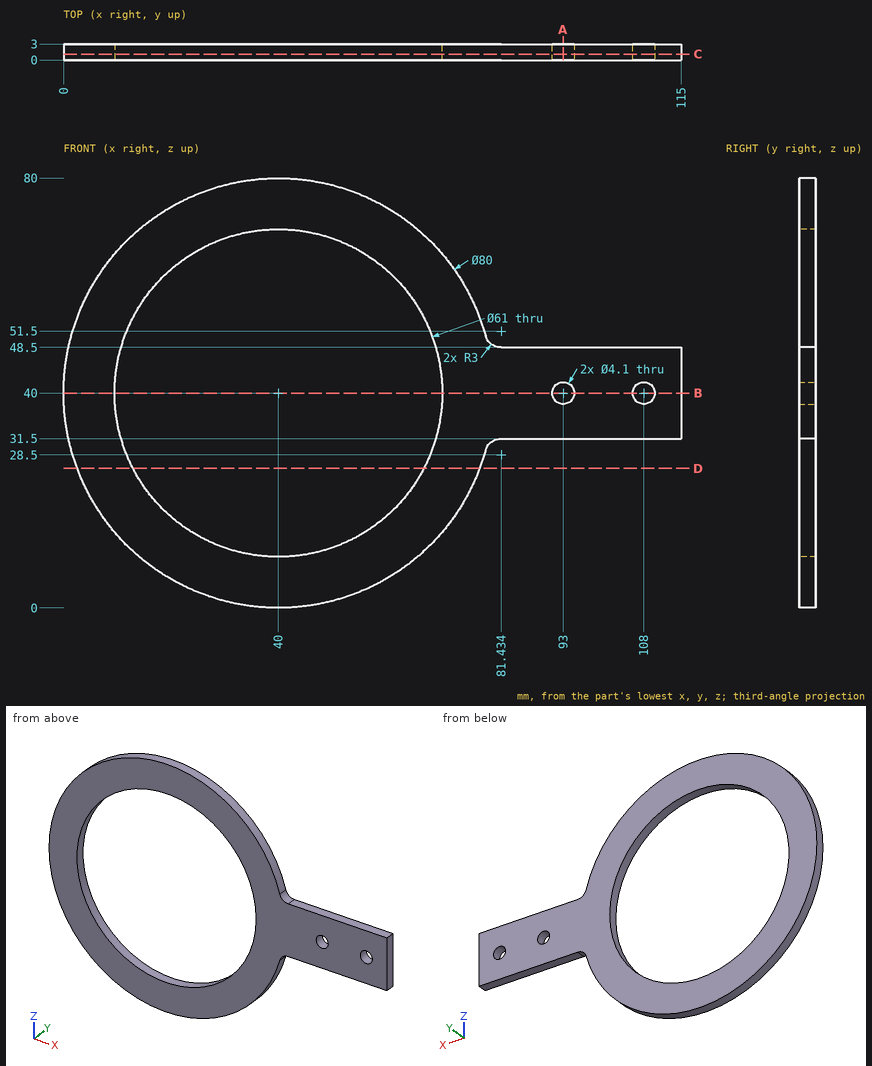
Input: dimensioned drawing with shaded views. Units: mm. Origin: part minimum x, y, z. Coordinates: 2 decimals unless noted, no trailing zeros. Loops run counter-clockwise (first coordinate to the right, second up) from the corner with the lowest first, then second, coordinate; pieces in that order, holes last. Notation, with made-up numbers: (-15, 78) -> (5, 78) arc R23 ccw to (5, 106) -> close; hole circle Ø8 at (-25, 13.5). An arc over 180 degrees is marked (long way). Use a Markdown table: item, result. Add a question column.
(1) Line query: line 1 along Z through (x, y) = (93, 1.75); line 2 along Z through (x, y) = (40, 2.3); line 3 along X through (y, z) = (0.55, 49.5) (1 decimal). Output: solid intervals per line, ascending.
(2) Section query A-A, the plane x = 93. Return loops of the section in (y, z), plus the area to 3 significant figures.
(3) Section query C-C, the plane y = 1.1. Return loops of the section in (x, z).
(4) Pin query (flat end, axial travel): pin 1 Ø1.5 at (x, y) = (23, 2) entering from -Z; pin 2 Ø0.9 at (x, y) = (101.5, 2) entering from -Z; pin 3 Ø4.5 at (x, z) = (93, 40) entering from -Y; pin 4 Ø2.5 at (x, z) = (108, 40) entering from -Y. Return the tip coordinate at first contact, or that it passes through.
(5) Section query B-B, the plane z = 40. Return loops of the section in (x, y), plus the area to 3 significant figures.
(6) Section query D-D, the plane z = 26. Return loops of the section in (x, y).
Answer:
| question | item | result |
|---|---|---|
| 1 | line 1 | z = 31.5 to 37.95, 42.05 to 48.5 |
| 1 | line 2 | z = 0 to 9.5, 70.5 to 80 |
| 1 | line 3 | x = 1.1 to 11, 69 to 79.2 |
| 2 | outline | (0, 31.5) -> (3, 31.5) -> (3, 37.95) -> (0, 37.95) -> close; (0, 42.05) -> (3, 42.05) -> (3, 48.5) -> (0, 48.5) -> close |
| 2 | area | 38.7 mm^2 |
| 3 | outline | (78.54, 29.3) arc R3 cw to (81.43, 31.5) -> (115, 31.5) -> (115, 48.5) -> (81.43, 48.5) arc R3 cw to (78.54, 50.7) arc R40 ccw (long way) to start; hole circle Ø61 at (40, 40); hole circle Ø4.1 at (93, 40); hole circle Ø4.1 at (108, 40) |
| 4 | pin 1 | stops at z = 3.45 |
| 4 | pin 2 | stops at z = 31.5 |
| 4 | pin 3 | stops at y = 0 |
| 4 | pin 4 | passes through |
| 5 | outline | (0, 0) -> (9.5, 0) -> (9.5, 3) -> (0, 3) -> close; (70.5, 0) -> (90.95, 0) -> (90.95, 3) -> (70.5, 3) -> close; (95.05, 0) -> (105.95, 0) -> (105.95, 3) -> (95.05, 3) -> close; (110.05, 0) -> (115, 0) -> (115, 3) -> (110.05, 3) -> close |
| 5 | area | 137 mm^2 |
| 6 | outline | (2.53, 0) -> (12.9, 0) -> (12.9, 3) -> (2.53, 3) -> close; (67.1, 0) -> (77.47, 0) -> (77.47, 3) -> (67.1, 3) -> close |
